```python
from build123d import *

# Parameters (mm, degrees)
F0_R     = 12.7
F1_DEPTH = 6.35
F2_R     = 7.231453
F3_DEPTH = 25.4
F4_R     = 3.608235
F5_DEPTH = 31.75
F6_R     = 0.508
F7_R     = 0.508
F8_R     = 0.508
F9_R     = 0.254


with BuildPart() as f1:
    # F0 (on Right) → F1 (new body)
    with BuildSketch(Plane.YZ):
        Circle(F0_R)
    extrude(amount=-F1_DEPTH)

    # F2 (on Right) → F3 (join)
    with BuildSketch(Plane.YZ):
        Circle(F2_R)
    extrude(amount=F3_DEPTH)

    # F4 (on face) → F5 (join)
    with BuildSketch(Plane.YZ.offset(25.4)):
        Circle(F4_R)
    extrude(amount=F5_DEPTH)

    # F6
    f6_edges = [f1.edges().sort_by_distance(p)[0] for p in [
        (-6.35, -12.7, 0),
    ]]
    fillet(f6_edges, radius=F6_R)

    # F7
    f7_edges = [f1.edges().sort_by_distance(p)[0] for p in [
        (0, -12.7, 0),
    ]]
    fillet(f7_edges, radius=F7_R)

    # F8
    f8_edges = [f1.edges().sort_by_distance(p)[0] for p in [
        (25.4, -7.231453, 0),
    ]]
    fillet(f8_edges, radius=F8_R)

    # F9
    f9_edges = [f1.edges().sort_by_distance(p)[0] for p in [
        (57.15, -3.608235, 0),
    ]]
    fillet(f9_edges, radius=F9_R)


solid = f1.part
```
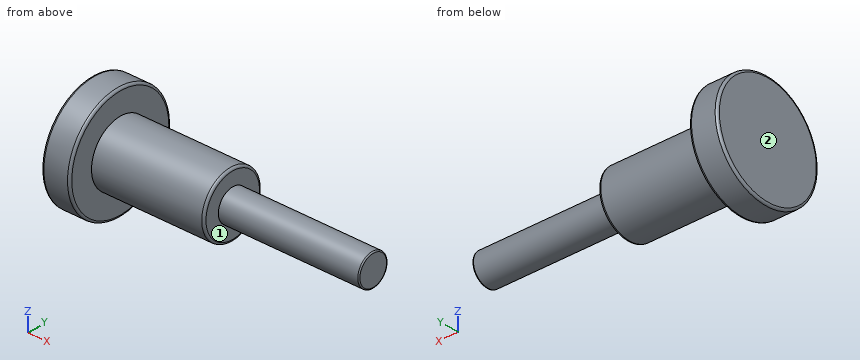
Build history of the part. All positions in model axes, mm. Face numbers are marked on the shaded views. A direction names the side the tool comes from. Give positions to 0.01 mm unless a question says otherwise; leave off trailing zeros. Loops run counter-clockwise (first coordinate to the right, second up) from the corner with the lowest first, then second, coordinate; pieces in that order, holes last. Notation, with made-up numbers: (2.25, 16) -> (7.25, 16) arc R16 cw to (7.25, 42) -> close; hole circle Ø11 at (63, 4.25). An arc over 180 degrees is marked (long way). One line per question, with ' | ' between items. Start each with the question number.
1) 3-axis set-ups, long thin cutter, end or side, ignore diameter. For the marked faces 1 and 2: which of +Z, -Z, +X, -X, +Y, -Y reach the whole face in a straight line?
2) Cut at D-D (x = 1). Give the cut face in (y, z).
3) Probe L1, parallel to X at y = 4.5, z = -3.25; L2, parallel to X at y = 5, z = -5.5; L3, parallel to Y at x = 29, z = 2.5. List the from-to ranges inside material, lowest first.
4) Cut at A-A (z = 0). Give the cut face in (x, y).
5) Pin check, flat tips, straight feed: pin 1 (12 mm diameter, centred on x = 13.5, z = -10, fed in from +Y); pin 2 (7.5 mm diameter, centred on y = 5.5, z = 5.5, fed in from +X); pin 3 (12 mm diameter, centred on x = 33.5, z = 6, fed in from +Y). Stop position of each tip, or through.
6) Cut at C-C (x = 50.5). Give the cut face in (y, z).
Return value:
1) face 1: +X | face 2: +Z, -Z, -X, +Y, -Y
2) outline: circle Ø14.46 at (0, 0)
3) L1: -6.35 to 25.4 | L2: -6.35 to 0 | L3: -2.6 to 2.6
4) outline: (-6.35, -12.19) arc R0.51 ccw to (-5.84, -12.7) -> (-0.51, -12.7) arc R0.51 ccw to (0, -12.19) -> (0, -7.23) -> (24.89, -7.23) arc R0.51 ccw to (25.4, -6.72) -> (25.4, -3.61) -> (56.9, -3.61) arc R0.25 ccw to (57.15, -3.35) -> (57.15, 3.35) arc R0.25 ccw to (56.9, 3.61) -> (25.4, 3.61) -> (25.4, 6.72) arc R0.51 ccw to (24.89, 7.23) -> (0, 7.23) -> (0, 12.19) arc R0.51 ccw to (-0.51, 12.7) -> (-5.84, 12.7) arc R0.51 ccw to (-6.35, 12.19) -> close
5) pin 1: y = 6.02 | pin 2: x = 25.4 | pin 3: y = 3.61
6) outline: circle Ø7.22 at (0, 0)
